```python
from build123d import *

# Parameters (mm, degrees)
F0_W     = 203.2
F0_H     = 508
F0_W_2   = 50.8
F0_H_2   = 152.4
F0_W_3   = 101.6
F0_H_3   = 101.6
F1_DEPTH = 50.8


with BuildPart() as f1:
    # F0 (on Front) → F1 (new body)
    with BuildSketch(Plane.XZ):
        with Locations((-977.9, -482.6)):
            Rectangle(F0_W, F0_H)
        with Locations((-977.9, -457.2)):
            Rectangle(F0_W_2, F0_H_2, mode=Mode.SUBTRACT)
        with Locations((977.9, -482.6)):
            Rectangle(F0_W, F0_H)
        with Locations((977.9, -457.2)):
            Rectangle(F0_W_2, F0_H_2, mode=Mode.SUBTRACT)
        with BuildLine():
            add(Edge.make_bspline(
                [(-1079.5, 228.6), (-968.1757741692, 184.2889311875), (-678.4073473646, 207.95738785), (-90.2517712986, 229.8963509513), (677.7555694837, 210.4033216408), (982.5995632946, 183.4544273595), (1079.5, 228.6)],
                knots=[0, 0, 0, 0, 0.2127647976, 0.4816607486, 0.7872352024, 1, 1, 1, 1], degree=3))
            Line((-1079.5, 228.6), (-1079.5, -228.6))
            Line((-1079.5, -228.6), (-876.3, -228.6))
            Line((-876.3, -228.6), (876.3, -228.6))
            Line((876.3, -228.6), (1079.5, -228.6))
            Line((1079.5, -228.6), (1079.5, 228.6))
        make_face()
        with Locations((-584.2, 76.2)):
            Rectangle(F0_W_3, F0_H_3, mode=Mode.SUBTRACT)
        with Locations((0, 76.2)):
            Rectangle(F0_W_3, F0_H_3, mode=Mode.SUBTRACT)
        with Locations((584.2, 76.2)):
            Rectangle(F0_W_3, F0_H_3, mode=Mode.SUBTRACT)
    extrude(amount=F1_DEPTH)


solid = f1.part
```
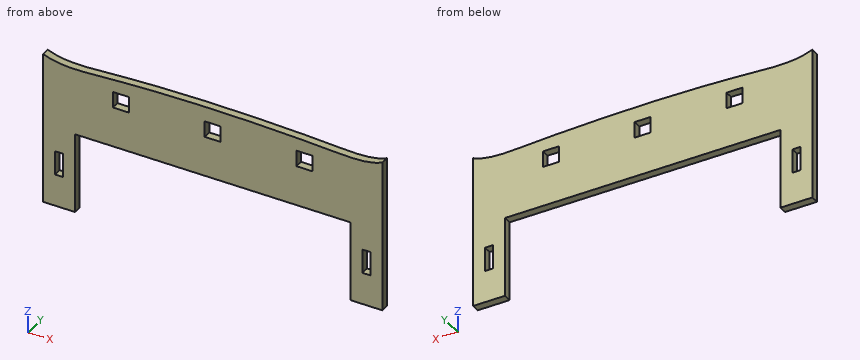
Source: CAD feature listing. Evaluate the final solid. Frame: model axes, mm. Give positions to 0.01 mm unless a question says otherwise; leave off trailing zeros. Write each loop counter-clockwise with the first axis right and the second up, starting at its lowest first coordinate (ties: lowest second). Pieces come first, ordered by that corner, then holes. Notation, with made-up numbers: (85, 55) - (101, 55) arc R22 cw to (101, 69) - close; hole circle Ø7 at (-34.5, 3). An arc over 180 degrees is marked (long way). One line per item, written item: value. Start each with the question number.
Q1. Section query A-A, the plane z = -646. Return the cut outline in (x, y), then the cut area to 3 significant figures.
Q2. Section query B-B, the plane z = -461.5. Return the cut outline in (x, y), then the cut area to 3 significant figures.
Q3. First-contact query: pin 1 Ø8 at (x, y) = (505, -13) entering from +Z; pin 2 Ø12 at (x, y) = (633.5, -23) entering from -Z. Flat tips, straight axial feed; report the tip coordinate or a pass-through.
Q4. Section query D-D, the plane z = 79.5. Return the cut outline in (x, y).
Q5. Material intervals for probe 1 along X at (y, z) = (-14, 113); probe 2 along X at (y, z) = (-2, -460.5); probe 3 along X at (y, z) = (-3.5, -559), sorted ascending. Write a range as from..to.
Q6. Section query C-C, the plane y = -31.5. Count the separate pieces of the cut face and the enclosed holes in it, then the cut area to 3 significant figures.
Answer:
1. outline: (-1079.5, -50.8) - (-876.3, -50.8) - (-876.3, 0) - (-1079.5, 0) - close; (876.3, -50.8) - (1079.5, -50.8) - (1079.5, 0) - (876.3, 0) - close
1. area: 20,600 mm2
2. outline: (-1079.5, -50.8) - (-1003.3, -50.8) - (-1003.3, 0) - (-1079.5, 0) - close; (-952.5, -50.8) - (-876.3, -50.8) - (-876.3, 0) - (-952.5, 0) - close; (876.3, -50.8) - (952.5, -50.8) - (952.5, 0) - (876.3, 0) - close; (1003.3, -50.8) - (1079.5, -50.8) - (1079.5, 0) - (1003.3, 0) - close
2. area: 15,500 mm2
3. pin 1: stops at z = 212.14
3. pin 2: stops at z = -228.6
4. outline: (-1079.5, -50.8) - (-635, -50.8) - (-635, 0) - (-1079.5, 0) - close; (-533.4, -50.8) - (-50.8, -50.8) - (-50.8, 0) - (-533.4, 0) - close; (50.8, -50.8) - (533.4, -50.8) - (533.4, 0) - (50.8, 0) - close; (635, -50.8) - (1079.5, -50.8) - (1079.5, 0) - (635, 0) - close
5. probe 1: x = -1079.5..-635, -533.4..-50.8, 50.8..533.4, 635..1079.5
5. probe 2: x = -1079.5..-1003.3, -952.5..-876.3, 876.3..952.5, 1003.3..1079.5
5. probe 3: x = -1079.5..-876.3, 876.3..1079.5
6. separate pieces: 1
6. enclosed holes: 5
6. area: 1,110,000 mm2
